Autodesk Inventor part; units mm, degrees
ref_plane "YZ Plane" through (0, 0, 0) normal (1, 0, 0) x (0, 1, 0)
ref_plane "XZ Plane" through (0, 0, 0) normal (0, 1, 0) x (-1, 0, 0)
ref_plane "XY Plane" through (0, 0, 0) normal (0, 0, 1) x (1, 0, 0)
sketch "Szkic1" plane through (0, 0, 0) normal (0, 1, 0) x (-1, 0, 0)
  line L0 (-4, 6.5) -> (4, 6.5) construction
  line L1 (4, 6.5) -> (4, -6.5) construction
  line L2 (4, -6.5) -> (-4, -6.5) construction
  line L3 (-4, -6.5) -> (-4, 6.5) construction
  line L4 (-4, 6.5) -> (4, -6.5) construction
  line L5 (4, 6.5) -> (-4, -6.5) construction
  line L6 (-5, -6.7) -> (5, -6.7)
  line L7 (5, -6.7) -> (5, 6.7)
  line L8 (5, 6.7) -> (-5, 6.7)
  line L9 (-5, 6.7) -> (-5, -6.7)
  line L10 (-5, -6.7) -> (5, 6.7) construction
  line L11 (5, -6.7) -> (-5, 6.7) construction
  line L12 (5, 6.7) -> (5, 11.7)
  line L13 (5, -6.7) -> (5, -11.7)
  line L14 (5, 11.7) -> (5, 14.7)
  line L15 (5, -11.7) -> (5, -14.7)
  line L16 (5, 14.7) -> (2, 14.7)
  line L17 (2, 14.7) -> (2, 11.7)
  line L18 (2, 11.7) -> (5, 11.7)
  line L19 (5, 11.7) -> (5, 14.7)
  line L20 (5, -14.7) -> (2, -14.7)
  line L21 (2, -14.7) -> (2, -11.7)
  line L22 (2, -11.7) -> (5, -11.7)
  line L23 (5, -11.7) -> (5, -14.7)
  line L24 (-5, 0) -> (-7, 0)
  line L25 (-5, 6.7) -> (-7, 6.7)
  line L26 (-5, -6.7) -> (-7, -6.7)
  line L27 (2, 11.7) -> (2, 8.7)
  line L28 (-7, 6.7) -> (-7, 0)
  line L29 (-7, 0) -> (-7, -6.7)
  line L30 (2, -11.7) -> (2, -8.7)
  line L31 (-5, 6.7) -> (-5, 8.7)
  line L32 (-5, 8.7) -> (2, 8.7)
  line L33 (-5, -6.7) -> (-5, -8.7)
  line L34 (-5, -8.7) -> (2, -8.7)
  line L35 (-5, 8.7) -> (-7, 6.7)
  line L36 (-7, -6.7) -> (-5, -8.7)
  point P0 (0, 0)
  dimension "d0" = 8
  dimension "d1" = 13
  dimension "d2" = 10
  dimension "d3" = 13.4
  dimension "d4" = 5
  dimension "d5" = 5
  dimension "d6" = 3
  dimension "d7" = 3
  dimension "d8" = 3
  dimension "d9" = 3
  dimension "d10" = 2
  dimension "d11" = 2
  dimension "d12" = 2
  dimension "d13" = 3
  dimension "d14" = 3
  dimension "d15" = 2
  dimension "d16" = 2
extrude "Wyciągnięcie proste1" add sketch "Szkic1" along normal blind 10 contours L26 L29 L24 L9 | L33 L36 L26 | L6 L13 L22 L30 L34 L33 | L24 L28 L25 L9 | L8 L31 L32 L27 L18 L12 | L15 L20 L21 L22 | L25 L35 L31 | L18 L17 L16 L14
sketch "Szkic2" plane through (-2, 0, 14.7) normal (1, 0, 0) x (0, 0, -1)
  line L0 (0, 10) -> (6, 10) construction
  line L1 (6, 0) -> (6, 10) construction
  line L2 (0, 0) -> (0, 10) construction
  line L3 (6, 0) -> (0, 0) construction
  line L4 (14.7, 0) -> (14.7, 10) construction
  line L5 (8, 10) -> (21.4, 10) construction
  circle A0 centre (3.2, 5) radius 1.5
  circle A1 centre (26.2, 5) radius 1.5
  line L6 (23.4, 0) -> (23.4, 10)
  line L7 (0, 0) -> (6, 10) construction
  line L8 (6, 0) -> (0, 10) construction
  line L9 (6, 0) -> (6, 10)
  point P0 (6, 5)
  point P1 (6, 5)
  dimension "d19" = 3
  dimension "d27" = 2.8
  dimension "d28" = 5
extrude "Wyciągnięcie proste2" cut sketch "Szkic2" against normal blind 6.65
fillet "Zaokrąglenie1" radius 2 4 edges at (-3.5, 10, 14.7) (-3.5, 0, 14.7) (-3.5, 10, -14.7) (-3.5, 0, -14.7)
properties part number "silnik_lockedin"
Model file for the job. Use its own axes, mm. A direction names the side the tool comes from. Give positions to 0.01 mm unless a question says otherwise; leave off trailing zeros. Order: outer loops, then holes, each group sorted by start corner. A loop starts at its lowest first (then second) coordinate and runs counter-clockwise, first axis right, second up. Notation, with made-up numbers: (-9.75, 74) -> (27.25, 74) arc R15 cw to (27.25, 102) -> close; hole circle Ø9 at (18.25, 50). An arc over 180 degrees is marked (long way). Use CSV: the item, a comma, the result in double quotes.
1. Band-saw the part on A-A, the plane x = -0.25. Give the cut face in (y, z).
Outcome:
outline,"(0, -8.7) -> (10, -8.7) -> (10, -6.7) -> (0, -6.7) -> close; (0, 6.7) -> (10, 6.7) -> (10, 8.7) -> (0, 8.7) -> close"
2. Drill centre lines: line 1 along Z through (x, y) = (3.75, 3.5); line 2 along X through (y, z) = (3.5, -12); line 3 along Y through (x, z) = (-3.1, -11.5). Where is each one in solid material? Low to high. Write a range as from..to.
Outcome:
line 1,"-8.7..-6.7, 6.7..8.7"
line 2,"-5..-2"
line 3,"0..3.5, 6.5..10"
3. Drop flat-ended pins along their axis: pin 1 (4 mm diameter, centred on x = 2.5, y = 8, fed in from -Z); pin 2 (5 mm diameter, centred on x = 4, z = -8.5, fed in from -Y); pin 3 (6 mm diameter, centred on x = 5.5, y = 6.5, fed in from +Z); pin 4 (2.5 mm diameter, centred on y = 5, z = 11.5, fed in from +X). Give the stop position or say it passes through.
Outcome:
pin 1,"z = -8.7"
pin 2,"y = 0"
pin 3,"z = 8.7"
pin 4,"through"
4. Mould opens along Z. For faces 4 (the cylindrical face through (-3.48, 0.6, 14.13)), 5 (the flat face through (0, 5, 6.7)), 6 (the flat face through (5.5, 0, 0.1)) say: +Z half, -Z half, draft (parallel to the pull), parting line (faces both ways), or undercut.
Outcome:
face 4,"+Z half"
face 5,"undercut"
face 6,"draft"
5. Band-saw the part on C-C, the plane z = -11.5. Give the cut face in (x, y), then the cut area to 3 significant figures.
Outcome:
outline,"(-5, 0) -> (-2, 0) -> (-2, 3.5) -> (-5, 3.5) -> close; (-5, 6.5) -> (-2, 6.5) -> (-2, 10) -> (-5, 10) -> close"
area,"21.0 mm²"
6. Band-saw the part on D-D, the plane y = 9.25. Give the cut face in (x, z), then the cut area to 3 significant figures.
Outcome:
outline,"(-5, -14.26) -> (-2, -14.26) -> (-2, -8.7) -> (5, -8.7) -> (7, -6.7) -> (7, 6.7) -> (5, 8.7) -> (-2, 8.7) -> (-2, 14.26) -> (-5, 14.26) -> (-5, 6.7) -> (5, 6.7) -> (5, -6.7) -> (-5, -6.7) -> close"
area,"104 mm²"
7. 3-axis set-ups, long thin cutter, end or side, ignore diameter. For faces 1 (the flat face through (-2, 4, 10)), 2 (the flat face through (2, 5, -8.7)), 3 (the flat face through (5, 5, 0)): which of +Z, -Z, +X, -X, +Y, -Y reach the whole face in a straight line?
Outcome:
face 1,"+Z, +X, +Y, -Y"
face 2,"-Z, +X, +Y, -Y"
face 3,"-X, +Y, -Y"
8. Band-saw the part on B-B, the plane y = 5. Give the cut face in (x, z), then the cut area to 3 significant figures.
Outcome:
outline,"(-5, -14.7) -> (-2, -14.7) -> (-2, -13) -> (-5, -13) -> close; (-5, -10) -> (-2, -10) -> (-2, -8.7) -> (5, -8.7) -> (7, -6.7) -> (7, 6.7) -> (5, 8.7) -> (-2, 8.7) -> (-2, 10) -> (-5, 10) -> (-5, 6.7) -> (5, 6.7) -> (5, -6.7) -> (-5, -6.7) -> close; (-5, 13) -> (-2, 13) -> (-2, 14.7) -> (-5, 14.7) -> close"
area,"88.8 mm²"
